from build123d import *

# Parameters (mm, degrees)
SKETCH1_R           = 3.5
BOSS_EXTRUDE1_DEPTH = 7
SKETCH3_W           = 45
SKETCH3_H           = 5.102229266
BOSS_EXTRUDE3_DEPTH = 35
FILLET2_R           = 5
FILLET6_R           = 5
SKETCH4_R           = 3.5
CUT_EXTRUDE1_DEPTH  = 5.102229266
SKETCH5_R           = 2.5
BOSS_EXTRUDE4_DEPTH = 10
SKETCH6_W           = 35
SKETCH6_H           = 5.102229266
BOSS_EXTRUDE5_DEPTH = 5
FILLET14_R          = 3
FILLET15_R          = 3
SKETCH7_R           = 0.75
CUT_EXTRUDE2_DEPTH  = 20


with BuildPart() as part:
    # Sketch1 → Boss-Extrude1 (new body)
    with BuildSketch(Plane.XY):
        with BuildLine():
            Line((-0.043255317, 12), (21.956744683, 12))
            Line((21.956744683, 12), (21.956744683, 7))
            ThreePointArc((21.956744683, 7), (13.877753218, -5.850552891), (-1.128e-06, -11.999922533))
            ThreePointArc((-1.128e-06, -11.999922533), (-12.000117541, -0.021549663), (-0.043255317, 12))
        make_face()
        with Locations((-0.000137029, 7.7466e-05)):
            Circle(SKETCH1_R, mode=Mode.SUBTRACT)
    extrude(amount=BOSS_EXTRUDE1_DEPTH)

    # Sketch3 → Boss-Extrude3 (add)
    with BuildSketch(Plane(origin=(21.956744683, 0, 0), x_dir=(0, 0, -1), z_dir=(1, 0, 0))):
        with Locations((-3.5, 9.5)):
            Rectangle(SKETCH3_W, SKETCH3_H)
    extrude(amount=BOSS_EXTRUDE3_DEPTH)

    # Fillet2
    fillet2_edges = [part.edges().sort_by_distance(p)[0] for p in [
        (21.956744683, 9.5, 0),
    ]]
    fillet(fillet2_edges, radius=FILLET2_R)

    # Fillet6
    fillet6_edges = [part.edges().sort_by_distance(p)[0] for p in [
        (21.956744683, 9.5, 7),
    ]]
    fillet(fillet6_edges, radius=FILLET6_R)

    # Sketch4 → Cut-Extrude1 (cut)
    with BuildSketch(Plane(origin=(0, 12.051114633, 0), x_dir=(1, 0, 0), z_dir=(0, 1, 0))):
        with Locations(Location((35.956744683, 7, 0), (0, 0, 180))):
            Circle(SKETCH4_R)
    extrude(amount=-CUT_EXTRUDE1_DEPTH, mode=Mode.SUBTRACT)

    # Sketch5 → Boss-Extrude4 (add)
    with BuildSketch(Plane(origin=(0, 12.051114633, 0), x_dir=(1, 0, 0), z_dir=(0, 1, 0))):
        with Locations((35.956744683, -20)):
            Circle(SKETCH5_R)
    extrude(amount=BOSS_EXTRUDE4_DEPTH)

    # Sketch6 → Boss-Extrude5 (add)
    with BuildSketch(Plane.XY.offset(26)):
        with Locations((39.456744683, 9.5)):
            Rectangle(SKETCH6_W, SKETCH6_H)
    extrude(amount=BOSS_EXTRUDE5_DEPTH)

    # Fillet14
    fillet14_edges = [part.edges().sort_by_distance(p)[0] for p in [
        (56.956744683, 9.5, -19),
    ]]
    fillet(fillet14_edges, radius=FILLET14_R)

    # Fillet15
    fillet15_edges = [part.edges().sort_by_distance(p)[0] for p in [
        (21.956744683, 9.5, -19),
        (21.956744683, 9.5, 31),
        (56.956744683, 9.5, 31),
    ]]
    fillet(fillet15_edges, radius=FILLET15_R)

    # Sketch7 → Cut-Extrude2 (cut)
    with BuildSketch(Plane.XY.offset(31)):
        with Locations((35.956744683, 19.051114633)):
            Circle(SKETCH7_R)
    extrude(amount=-CUT_EXTRUDE2_DEPTH, mode=Mode.SUBTRACT)


solid = part.part
Can you work these out from the model? Positions are in its coordinate system, mm. A direction names the side the tool comes from. Round coordinates to 2 decimals unless told otherwise and drop trailing zeros. Order: outer loops, then holes, each group sorted by start corner. A loop starts at its lowest first (then second) coordinate and runs counter-clockwise, first axis right, second up. Notation, with made-up numbers: (-16, -26) -> (9, -26) arc R31 cw to (9, 10) -> close; hole circle Ø7 at (47, 55). An arc over 180 degrees is marked (long way). Write each question's results on one line, items separated by ' | '. Start each with the question number.
Item 1: Will these pins go through, and if not, where does the flat tip stop? pin 1 (12 mm diameter, centred on x = 33, z = 22, fed in from +Y); pin 2 (4 mm diameter, centred on y = 10.5, z = 11, fed in from -X); pin 3 (7 mm diameter, centred on x = 2.5, y = 5.5, fed in from +Z); pin 4 (2 mm diameter, centred on x = 35.96, y = 19.05, fed in from +Z).
Item 2: Which directions (+Z, -Z, +X, -X, +Y, -Y) give clear straight access to the entire face, cutting with the end or side of a thin tool? Please do faces 1 (the cylindrical face through (38.34, 16.98, 19.25)), 2 (the flat face through (36, 22.051, 20)), 3 (the flat face through (39, 6.949, 6)).
Item 3: Thinking about a two-plate mould opening in Z: for faces 4 (the flat face through (39, 10, 31)), 5 (the cylindrical face through (39.453, 9.536, -6.846)), 6 (the flat face through (3, 3, 0)), which applies, +Z half, -Z half, draft (parallel to the pull), parting line (faces both ways), or undercut?
Item 4: If we section it at D-D, the plane x = 26: Write out the boundary of the cut face in (y, z), then the cut area to 3 significant figures.
Item 5: If we section it at A-A, the plane z = -7: Write out the boundary of the cut face in (x, y).
Item 6: If we section it at B-B, the plane y = 10.5: Write out the boundary of the cut face in (x, z).
Item 7: Please list where these lines run through material, in increasing order: L1, parallel to Y at x = 41, z = 25; L2, parallel to Z at x = -2, y = 5.5; L3, parallel to X at y = -10, z = 4.
Item 8: If we section it at C-C, the plane z = 21: Write out the boundary of the cut face in (x, y).
Results:
1) pin 1: stops at y = 22.05 | pin 2: stops at x = 20.96 | pin 3: stops at z = 7 | pin 4: stops at z = 22.5
2) face 1: +Y | face 2: +Z, -Z, +X, -X, +Y | face 3: +Z, -Z, +X, -Y
3) face 4: +Z half | face 5: undercut | face 6: -Z half
4) outline: (6.95, -19) -> (12.05, -19) -> (12.05, 31) -> (6.95, 31) -> close | area: 255 mm2
5) outline: (21.96, 6.95) -> (32.46, 6.95) -> (32.46, 12.05) -> (21.96, 12.05) -> close; (39.46, 6.95) -> (56.96, 6.95) -> (56.96, 12.05) -> (39.46, 12.05) -> close
6) outline: (-5.81, 0) -> (16.96, 0) arc R5 cw to (21.96, -5) -> (21.96, -16) arc R3 ccw to (24.96, -19) -> (53.96, -19) arc R3 ccw to (56.96, -16) -> (56.96, 28) arc R3 ccw to (53.96, 31) -> (24.96, 31) arc R3 ccw to (21.96, 28) -> (21.96, 12) arc R5 cw to (16.96, 7) -> (-5.81, 7) -> close; hole circle Ø7 at (35.96, -7)
7) L1: y = 6.95 to 12.05 | L2: z = 0 to 7 | L3: x = -6.63 to 7.31
8) outline: (21.96, 6.95) -> (56.96, 6.95) -> (56.96, 12.05) -> (38.25, 12.05) -> (38.25, 22.05) -> (33.67, 22.05) -> (33.67, 12.05) -> (21.96, 12.05) -> close; hole circle Ø1.5 at (35.96, 19.05)
